The figure shows three views and two pictorial views of one solid part (mm, origin at its lowest corner). Answer the questions. Give positions to 0.01 mm unless a question says otherwise; leave off trailing zeros. Order: outer loops, then holes, each group sorted by start corner. A loop starts at its lowest first (then second) coordinate and runs counter-clockwise, first axis right, second up. Notation, with made-up numbers: (17, -30.75) - (72, -30.75) arc R31 cw to (72, -2.75) - close; hole circle Ø10 at (-36.75, 50.25). An arc over 180 degrees is marked (long way). Use a Markdown table: item, result. Add a question column.
1. For a pull along Z with two mould halves and no side action, classify the marked faces 1, 2 and 3 as released by +Z, released by -Z, zero draft, split by the parting line, or undercut.
2. Consider L1, parallel to Z at x = 22.25, y = 42 (1 decimal); L2, parallel to Y at x = 24, z = 7 (1 decimal); L3, parallel to Z at x = 13, y = 50 (1 decimal). Determine where each line is inside the solid, lowest interval first.
3. A cutting plane is placed at D-D on y = 5. Determine the outline of the cut face in (x, z).
4. Flat-ended cylindrical pins translate along their axes: P1, Ø5, axis at x = 16.5, z = 38, coming from the +Y side; P2, Ø10, axis at y = 18, z = 48, coming from the -X side; P3, Ø8, axis at x = 9.5, z = 18, coming from the -Y side. Find the tip coordinate at first contact, or state that the pin passes through.
5. A cutting plane is placed at A-A on y = 53. Determine the outline of the cut face in (x, z).
6. A cutting plane is placed at B-B on z = 32.5. Determine the outline of the cut face in (x, y) (1 decimal), and give its area (3 significant figures).
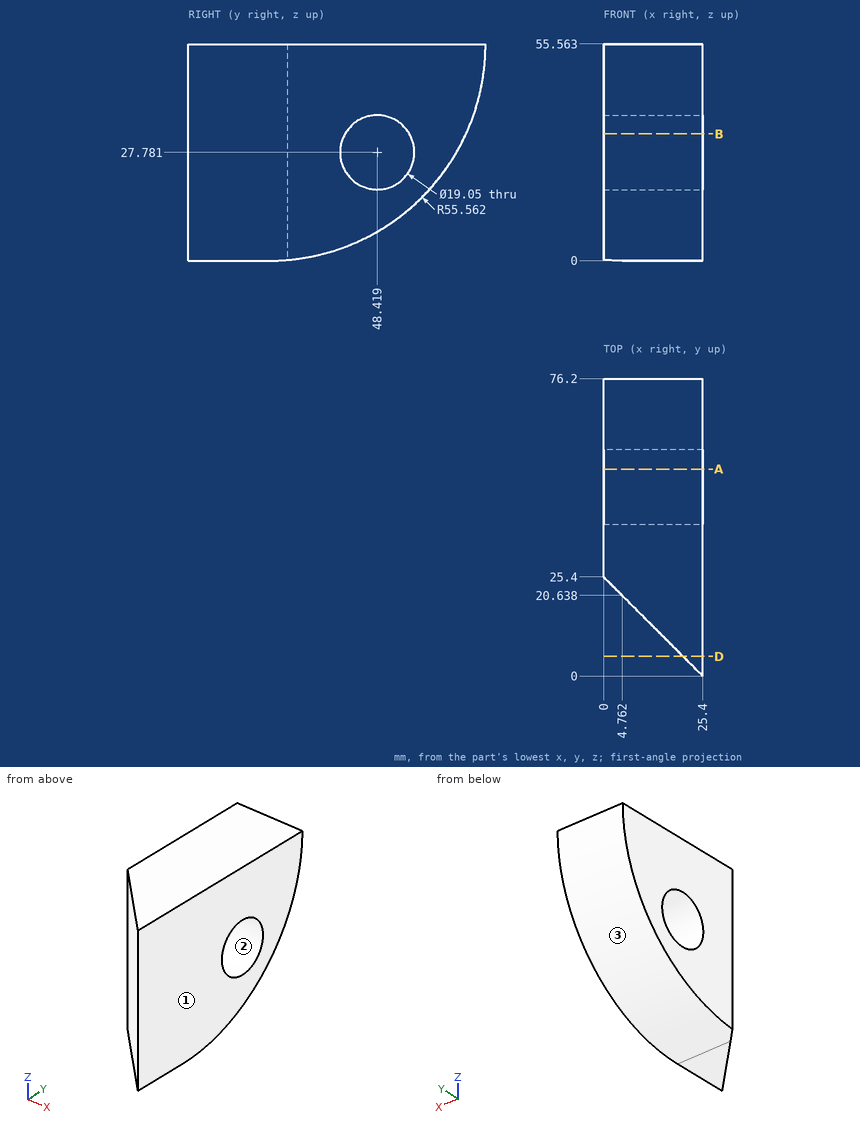
Output values:
| question | item | result |
|---|---|---|
| 1 | face 1 | zero draft |
| 1 | face 2 | undercut |
| 1 | face 3 | released by -Z |
| 2 | L1 | 4.3 to 20.7, 34.8 to 55.6 |
| 2 | L2 | 1.4 to 47.6 |
| 2 | L3 | 8.4 to 18.4, 37.2 to 55.6 |
| 3 | outline | (20.4, 0) - (25.4, 0) - (25.4, 55.56) - (20.4, 55.56) - close |
| 4 | P1 | y = 74.12 |
| 4 | P2 | x = 2.4 |
| 4 | P3 | y = 11.9 |
| 5 | outline | (0, 10.4) - (25.4, 10.4) - (25.4, 19.43) - (0, 19.43) - close; (0, 36.13) - (25.4, 36.13) - (25.4, 55.56) - (0, 55.56) - close |
| 6 | outline | (0, 25.4) - (25.4, 0) - (25.4, 40.1) - (0, 40.1) - close; (0, 56.7) - (25.4, 56.7) - (25.4, 71.2) - (0, 71.2) - close |
| 6 | area | 1,070 mm² |
